Job drawing, mm, ordinate dimensions from the low corner. One solid piece. A direction names the side the tool comes from. Give positions to 0.01 mm unless a question says otherwise; leave off trailing zeros. Order: outer loops, then holes, each group sorted by start corner. A loop starts at its lowest first (then second) coordinate and runs counter-clockwise, first axis right, second up. Notation, with made-up numbers: M 88,-28.5 L 141,-28.5 A26 cw 141,0.5 Z; hole C 0.25,6.5 d1. An arc over 180 degrees is marked long. One line per item, written item: value. Start each with the question number.
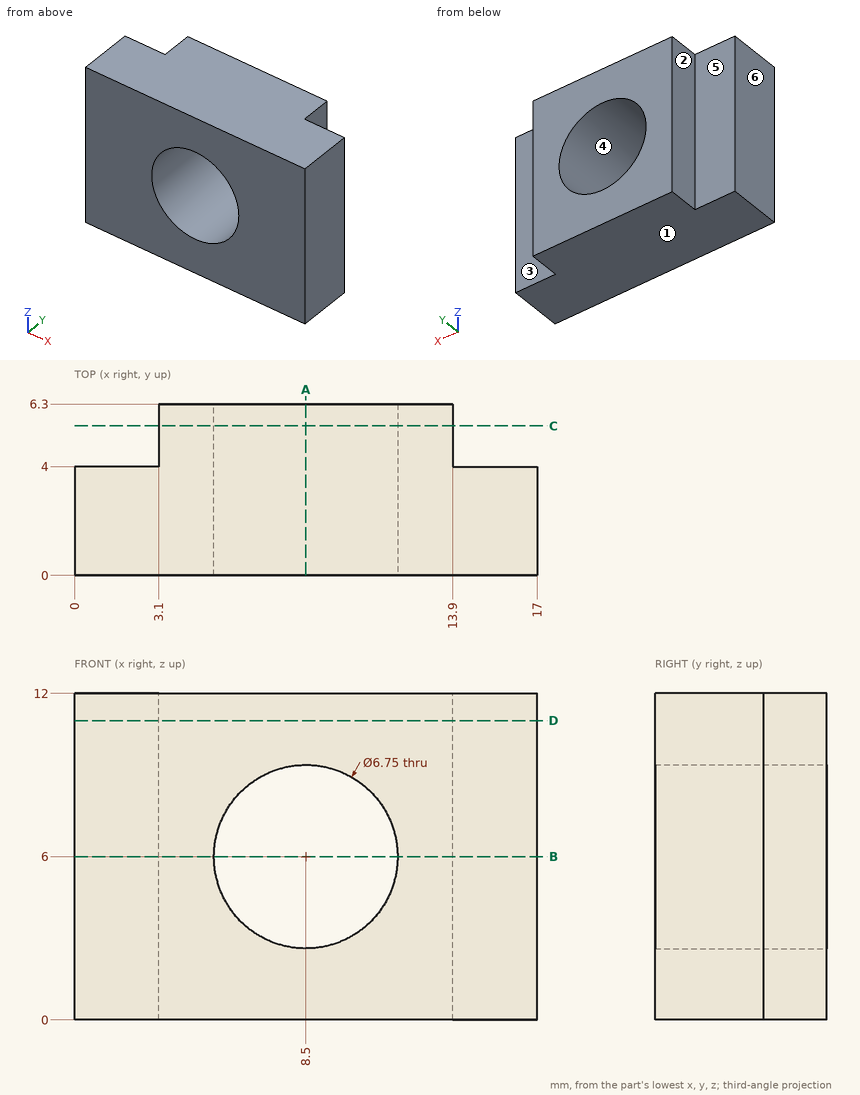
1) Slice it at C-C (y = 5.5). List the corners of the cut face in (x, z) (3 decimals).
2) Drop flat-ended pins along their axis: P1, Ø0.7, axis at y = 5, z = 6.5, coming from the +X side; P2, Ø0.9, axis at x = 15.5, z = 3.5, coming from the +Y side; P3, Ø1.2, axis at y = 5.5, z = 4.5, coming from the -X side. Give the stop position or say it passes through.
3) Slice it at A-A (x = 8.5). List the corners of the cut face in (y, z) (3 decimals), plus the area to 3 significant figures.
4) Drill centre lines: line 1 (Z direction, x = 8.5, y = 1.5) (3 decimals); line 2 (X direction, y = 2.75, z = 6) (3 decimals); line 3 (X direction, y = 5.5, z = 6) (3 decimals). Where is each one in solid material? Low to high.
5) Slice it at B-B (z = 6). List the corners of the cut face in (x, y) (3 decimals), plus the area to 3 significant figures.
6) Slice it at D-D (z = 11). List the corners of the cut face in (x, y).
7) Tool access for the marked faces 1, 2 and 3: list every direction of +Z, -Z, +X, -X, +Y, -Y with a clear straight run to the whole face (end or side of a thin tool).
8) Pull direction X, two halves, no side cores. Call the marked faces 4, 5 and 6: pulls with the +X half, pulls with the -X half, needs draft (parallel to the pull), parting line crosses it, or undercut.
Results list:
1. outline: M 3.1,0 L 13.9,0 L 13.9,12 L 3.1,12 Z; hole C 8.5,6 d6.75
2. P1: stops at x = 13.9
2. P2: stops at y = 4
2. P3: stops at x = 3.1
3. outline: M 0,0 L 6.3,0 L 6.3,2.625 L 0,2.625 Z; M 0,9.375 L 6.3,9.375 L 6.3,12 L 0,12 Z
3. area: 33.1 mm²
4. line 1: z = 0 to 2.625, 9.375 to 12
4. line 2: x = 0 to 5.125, 11.875 to 17
4. line 3: x = 3.1 to 5.125, 11.875 to 13.9
5. outline: M 0,0 L 5.125,0 L 5.125,6.3 L 3.1,6.3 L 3.1,4 L 0,4 Z; M 11.875,0 L 17,0 L 17,4 L 13.9,4 L 13.9,6.3 L 11.875,6.3 Z
5. area: 50.3 mm²
6. outline: M 0,0 L 17,0 L 17,4 L 13.9,4 L 13.9,6.3 L 3.1,6.3 L 3.1,4 L 0,4 Z
7. face 1: -Z, +X, -X, +Y, -Y
7. face 2: +Z, -Z, -X, +Y
7. face 3: +Z, -Z, +X, +Y
8. face 4: undercut
8. face 5: needs draft
8. face 6: pulls with the -X half
